Work out the finished part from the listing and answer in its coordinate system (mm). Coordinates: 2 decimals unless noted, no trailing zeros. Order: outer loops, then holes, each group sorted by start corner. A loop starts at its lowest first (then second) coordinate and runs counter-clockwise, first axis right, second up. Notation, with made-up numbers: M 42.5,45.25 L 80.5,45.25 A32 ccw 80.5,73.25 Z; hole C 39,29 d7. An arc over 180 degrees is marked long. Use a Markdown table: item, result.
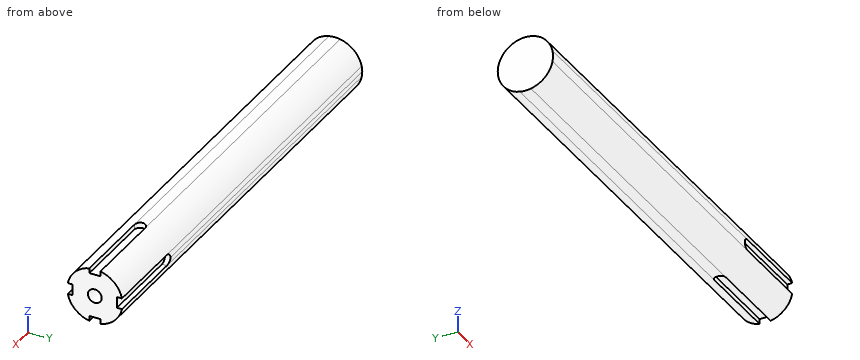
from build123d import *

# Parameters (mm, degrees)
F0_W      = 4
F0_H      = 4
F1_DEPTH  = 30
F2_DEPTH  = 130
F3_R      = 2
F4_DEPTH  = 25
F5_R      = 2
F6_DEPTH  = 25
F7_R      = 2
F8_DEPTH  = 25
F9_R      = 2
F10_DEPTH = 25
F12_D     = 5
F12_DEPTH = 20
F12_TIP   = 1.5021515476


with BuildPart() as f1:
    # F0 (on Right) → F1 (new body)
    with BuildSketch(Plane.YZ):
        with BuildLine():
            ThreePointArc((2, 7.2284161474), (5.3033008589, 5.3033008589), (7.2284161474, 2))
            Line((7.2284161474, 2), (8, 2))
            Line((8, 2), (9.7979589711, 2))
            ThreePointArc((9.7979589711, 2), (7.0710678119, 7.0710678119), (2, 9.7979589711))
            Line((2, 9.7979589711), (2, 8))
            Line((2, 8), (2, 7.2284161474))
        make_face()
        with BuildLine():
            ThreePointArc((-7.2284161474, 2), (-5.3033008589, 5.3033008589), (-2, 7.2284161474))
            Line((-2, 7.2284161474), (-2, 8))
            Line((-2, 8), (-2, 9.7979589711))
            ThreePointArc((-2, 9.7979589711), (-7.0710678119, 7.0710678119), (-9.7979589711, 2))
            Line((-9.7979589711, 2), (-8, 2))
            Line((-8, 2), (-7.2284161474, 2))
        make_face()
        with BuildLine():
            Line((2, 2), (7.2284161474, 2))
            ThreePointArc((7.2284161474, 2), (5.3033008589, 5.3033008589), (2, 7.2284161474))
            Line((2, 7.2284161474), (2, 2))
        make_face()
        with BuildLine():
            Line((2, 2), (2, 7.2284161474))
            ThreePointArc((2, 7.2284161474), (0, 7.5), (-2, 7.2284161474))
            Line((-2, 7.2284161474), (-2, 2))
            Line((-2, 2), (2, 2))
        make_face()
        with BuildLine():
            Line((-2, 2), (-2, 7.2284161474))
            ThreePointArc((-2, 7.2284161474), (-5.3033008589, 5.3033008589), (-7.2284161474, 2))
            Line((-7.2284161474, 2), (-2, 2))
        make_face()
        with BuildLine():
            Line((-2, -2), (-2, 2))
            Line((-2, 2), (-7.2284161474, 2))
            ThreePointArc((-7.2284161474, 2), (-7.5, 0), (-7.2284161474, -2))
            Line((-7.2284161474, -2), (-2, -2))
        make_face()
        with BuildLine():
            ThreePointArc((7.2284161474, -2), (7.4317938987, -1.0091776094), (7.5, 0))
            ThreePointArc((7.5, 0), (7.4317938987, 1.0091776094), (7.2284161474, 2))
            Line((7.2284161474, 2), (2, 2))
            Line((2, 2), (2, -2))
            Line((2, -2), (7.2284161474, -2))
        make_face()
        Rectangle(F0_W, F0_H)
        with BuildLine():
            ThreePointArc((-2, -7.2284161474), (0, -7.5), (2, -7.2284161474))
            Line((2, -7.2284161474), (2, -2))
            Line((2, -2), (-2, -2))
            Line((-2, -2), (-2, -7.2284161474))
        make_face()
        with BuildLine():
            ThreePointArc((-7.2284161474, -2), (-5.3033008589, -5.3033008589), (-2, -7.2284161474))
            Line((-2, -7.2284161474), (-2, -2))
            Line((-2, -2), (-7.2284161474, -2))
        make_face()
        with BuildLine():
            ThreePointArc((2, -7.2284161474), (5.3033008589, -5.3033008589), (7.2284161474, -2))
            Line((7.2284161474, -2), (2, -2))
            Line((2, -2), (2, -7.2284161474))
        make_face()
        with BuildLine():
            Line((8, -2), (7.2284161474, -2))
            ThreePointArc((7.2284161474, -2), (5.3033008589, -5.3033008589), (2, -7.2284161474))
            Line((2, -7.2284161474), (2, -8))
            Line((2, -8), (2, -9.7979589711))
            ThreePointArc((2, -9.7979589711), (7.0710678119, -7.0710678119), (9.7979589711, -2))
            Line((9.7979589711, -2), (8, -2))
        make_face()
        with BuildLine():
            Line((-2, -8), (-2, -7.2284161474))
            ThreePointArc((-2, -7.2284161474), (-5.3033008589, -5.3033008589), (-7.2284161474, -2))
            Line((-7.2284161474, -2), (-8, -2))
            Line((-8, -2), (-9.7979589711, -2))
            ThreePointArc((-9.7979589711, -2), (-7.0710678119, -7.0710678119), (-2, -9.7979589711))
            Line((-2, -9.7979589711), (-2, -8))
        make_face()
        with BuildLine():
            Line((2, -8), (2, -7.2284161474))
            ThreePointArc((2, -7.2284161474), (0, -7.5), (-2, -7.2284161474))
            Line((-2, -7.2284161474), (-2, -8))
            Line((-2, -8), (2, -8))
        make_face()
        with BuildLine():
            ThreePointArc((7.2284161474, 2), (7.4317938987, 1.0091776094), (7.5, 0))
            ThreePointArc((7.5, 0), (7.4317938987, -1.0091776094), (7.2284161474, -2))
            Line((7.2284161474, -2), (8, -2))
            Line((8, -2), (8, 2))
            Line((8, 2), (7.2284161474, 2))
        make_face()
        with BuildLine():
            ThreePointArc((-2, 7.2284161474), (0, 7.5), (2, 7.2284161474))
            Line((2, 7.2284161474), (2, 8))
            Line((2, 8), (-2, 8))
            Line((-2, 8), (-2, 7.2284161474))
        make_face()
        with BuildLine():
            ThreePointArc((-7.2284161474, -2), (-7.5, 0), (-7.2284161474, 2))
            Line((-7.2284161474, 2), (-8, 2))
            Line((-8, 2), (-8, -2))
            Line((-8, -2), (-7.2284161474, -2))
        make_face()
    extrude(amount=F1_DEPTH)

    # F0 (on Right) → F2 (join)
    with BuildSketch(Plane.YZ):
        with BuildLine():
            Line((-2, 8), (2, 8))
            Line((2, 8), (2, 9.7979589711))
            ThreePointArc((2, 9.7979589711), (0, 10), (-2, 9.7979589711))
            Line((-2, 9.7979589711), (-2, 8))
        make_face()
        with BuildLine():
            ThreePointArc((2, 7.2284161474), (5.3033008589, 5.3033008589), (7.2284161474, 2))
            Line((7.2284161474, 2), (8, 2))
            Line((8, 2), (9.7979589711, 2))
            ThreePointArc((9.7979589711, 2), (7.0710678119, 7.0710678119), (2, 9.7979589711))
            Line((2, 9.7979589711), (2, 8))
            Line((2, 8), (2, 7.2284161474))
        make_face()
        with BuildLine():
            ThreePointArc((-2, 7.2284161474), (0, 7.5), (2, 7.2284161474))
            Line((2, 7.2284161474), (2, 8))
            Line((2, 8), (-2, 8))
            Line((-2, 8), (-2, 7.2284161474))
        make_face()
        with BuildLine():
            ThreePointArc((-7.2284161474, 2), (-5.3033008589, 5.3033008589), (-2, 7.2284161474))
            Line((-2, 7.2284161474), (-2, 8))
            Line((-2, 8), (-2, 9.7979589711))
            ThreePointArc((-2, 9.7979589711), (-7.0710678119, 7.0710678119), (-9.7979589711, 2))
            Line((-9.7979589711, 2), (-8, 2))
            Line((-8, 2), (-7.2284161474, 2))
        make_face()
        with BuildLine():
            ThreePointArc((-7.2284161474, -2), (-7.5, 0), (-7.2284161474, 2))
            Line((-7.2284161474, 2), (-8, 2))
            Line((-8, 2), (-8, -2))
            Line((-8, -2), (-7.2284161474, -2))
        make_face()
        with BuildLine():
            Line((-8, -2), (-8, 2))
            Line((-8, 2), (-9.7979589711, 2))
            ThreePointArc((-9.7979589711, 2), (-10, 0), (-9.7979589711, -2))
            Line((-9.7979589711, -2), (-8, -2))
        make_face()
        with BuildLine():
            Line((-2, 2), (-2, 7.2284161474))
            ThreePointArc((-2, 7.2284161474), (-5.3033008589, 5.3033008589), (-7.2284161474, 2))
            Line((-7.2284161474, 2), (-2, 2))
        make_face()
        with BuildLine():
            Line((2, 2), (2, 7.2284161474))
            ThreePointArc((2, 7.2284161474), (0, 7.5), (-2, 7.2284161474))
            Line((-2, 7.2284161474), (-2, 2))
            Line((-2, 2), (2, 2))
        make_face()
        with BuildLine():
            Line((2, 2), (7.2284161474, 2))
            ThreePointArc((7.2284161474, 2), (5.3033008589, 5.3033008589), (2, 7.2284161474))
            Line((2, 7.2284161474), (2, 2))
        make_face()
        with BuildLine():
            Line((9.7979589711, 2), (8, 2))
            Line((8, 2), (8, -2))
            Line((8, -2), (9.7979589711, -2))
            ThreePointArc((9.7979589711, -2), (9.9493615301, -1.0050896201), (10, 0))
            ThreePointArc((10, 0), (9.9493615301, 1.0050896201), (9.7979589711, 2))
        make_face()
        with BuildLine():
            ThreePointArc((7.2284161474, 2), (7.4317938987, 1.0091776094), (7.5, 0))
            ThreePointArc((7.5, 0), (7.4317938987, -1.0091776094), (7.2284161474, -2))
            Line((7.2284161474, -2), (8, -2))
            Line((8, -2), (8, 2))
            Line((8, 2), (7.2284161474, 2))
        make_face()
        with BuildLine():
            ThreePointArc((7.2284161474, -2), (7.4317938987, -1.0091776094), (7.5, 0))
            ThreePointArc((7.5, 0), (7.4317938987, 1.0091776094), (7.2284161474, 2))
            Line((7.2284161474, 2), (2, 2))
            Line((2, 2), (2, -2))
            Line((2, -2), (7.2284161474, -2))
        make_face()
        Rectangle(F0_W, F0_H)
        with BuildLine():
            Line((-2, -2), (-2, 2))
            Line((-2, 2), (-7.2284161474, 2))
            ThreePointArc((-7.2284161474, 2), (-7.5, 0), (-7.2284161474, -2))
            Line((-7.2284161474, -2), (-2, -2))
        make_face()
        with BuildLine():
            ThreePointArc((-7.2284161474, -2), (-5.3033008589, -5.3033008589), (-2, -7.2284161474))
            Line((-2, -7.2284161474), (-2, -2))
            Line((-2, -2), (-7.2284161474, -2))
        make_face()
        with BuildLine():
            Line((-2, -8), (-2, -7.2284161474))
            ThreePointArc((-2, -7.2284161474), (-5.3033008589, -5.3033008589), (-7.2284161474, -2))
            Line((-7.2284161474, -2), (-8, -2))
            Line((-8, -2), (-9.7979589711, -2))
            ThreePointArc((-9.7979589711, -2), (-7.0710678119, -7.0710678119), (-2, -9.7979589711))
            Line((-2, -9.7979589711), (-2, -8))
        make_face()
        with BuildLine():
            Line((2, -8), (2, -7.2284161474))
            ThreePointArc((2, -7.2284161474), (0, -7.5), (-2, -7.2284161474))
            Line((-2, -7.2284161474), (-2, -8))
            Line((-2, -8), (2, -8))
        make_face()
        with BuildLine():
            Line((2, -9.7979589711), (2, -8))
            Line((2, -8), (-2, -8))
            Line((-2, -8), (-2, -9.7979589711))
            ThreePointArc((-2, -9.7979589711), (0, -10), (2, -9.7979589711))
        make_face()
        with BuildLine():
            ThreePointArc((2, -7.2284161474), (5.3033008589, -5.3033008589), (7.2284161474, -2))
            Line((7.2284161474, -2), (2, -2))
            Line((2, -2), (2, -7.2284161474))
        make_face()
        with BuildLine():
            Line((8, -2), (7.2284161474, -2))
            ThreePointArc((7.2284161474, -2), (5.3033008589, -5.3033008589), (2, -7.2284161474))
            Line((2, -7.2284161474), (2, -8))
            Line((2, -8), (2, -9.7979589711))
            ThreePointArc((2, -9.7979589711), (7.0710678119, -7.0710678119), (9.7979589711, -2))
            Line((9.7979589711, -2), (8, -2))
        make_face()
        with BuildLine():
            ThreePointArc((-2, -7.2284161474), (0, -7.5), (2, -7.2284161474))
            Line((2, -7.2284161474), (2, -2))
            Line((2, -2), (-2, -2))
            Line((-2, -2), (-2, -7.2284161474))
        make_face()
    extrude(amount=-F2_DEPTH)

    # F3 (on face) → F4 (cut)
    with BuildSketch(Plane.XY.offset(8)):
        Circle(F3_R)
    extrude(amount=F4_DEPTH, mode=Mode.SUBTRACT)

    # F5 (on face) → F6 (cut)
    with BuildSketch(Plane.XZ.offset(8)):
        Circle(F5_R)
    extrude(amount=F6_DEPTH, mode=Mode.SUBTRACT)

    # F7 (on face) → F8 (cut)
    with BuildSketch(Plane(origin=(0, 0, -8), x_dir=(1, 0, 0), z_dir=(0, 0, -1))):
        Circle(F7_R)
    extrude(amount=F8_DEPTH, mode=Mode.SUBTRACT)

    # F9 (on face) → F10 (cut)
    with BuildSketch(Plane(origin=(0, 8, 0), x_dir=(-1, 0, 0), z_dir=(0, 1, 0))):
        Circle(F9_R)
    extrude(amount=F10_DEPTH, mode=Mode.SUBTRACT)

    # F12
    with Locations(Plane.YZ.offset(30)):
        with Locations((0, 0)):
            Hole(F12_D / 2, depth=F12_DEPTH)
            with Locations((0, 0, -(F12_DEPTH + F12_TIP / 2))):  # 118° drill point
                Cone(0, F12_D / 2, F12_TIP, mode=Mode.SUBTRACT)


solid = f1.part
(1) A cutting plane is placed at A-A (x = -6). Determine the outline of the cut face in (y, z), then the cut area to 3 significant figures.
Conclusion:
| item | result |
|---|---|
| outline | C 0,0 d20 |
| area | 314 mm2 |
(2) Straight lines are drawn through the part: L1, parallel to Z at x = 19.5, y = 0; L2, parallel to Y at x = -116, z = 0.5. For each, find the intervals that lie inside material, in ascending order.
Conclusion:
| item | result |
|---|---|
| L1 | -8 to -2.5, 2.5 to 8 |
| L2 | -9.99 to 9.99 |
(3) A cutting plane is placed at B-B (y = -4.75). Determine the outline of the cut face in (x, z), then the cut area to 3 significant figures.
Conclusion:
| item | result |
|---|---|
| outline | M -130,-8.8 L 30,-8.8 L 30,8.8 L -130,8.8 Z |
| area | 2,820 mm2 |
(4) Given P1, Ø2, axis at x = 1, z = -4.5, coming from the +Y side; P2, Ø1.4, axis at x = 10, y = 9.5, coming from the +Z side; P3, Ø0.5, axis at x = 10.5, y = -8.5, coming from the -Z side; P4, Ø10, axis at x = -61, z = -1, coming from the +Y side, each flat-ended and moving along its own axis, determine where each tip first touches the part or whether it passes through.
Conclusion:
| item | result |
|---|---|
| P1 | y = 9.37 |
| P2 | z = 4.75 |
| P3 | z = -5.65 |
| P4 | y = 10 |
